from build123d import *

# Parameters (mm, degrees)
F0_W     = 12.85
F0_H     = 12.85
F0_W_2   = 6.2
F0_H_2   = 6.2
F1_DEPTH = 25
F2_DEPTH = 32.35
F3_SIZE  = 0.5
F4_SIZE  = 1


with BuildPart() as f1:
    # F0 (on Top) → F1 (new body)
    with BuildSketch(Plane.XY):
        Rectangle(F0_W, F0_H)
        Rectangle(F0_W_2, F0_H_2, mode=Mode.SUBTRACT)
    extrude(amount=F1_DEPTH)

    # F0 (on Top) → F2 (join)
    with BuildSketch(Plane.XY):
        Rectangle(F0_W_2, F0_H_2)
    extrude(amount=F2_DEPTH)

    # F3
    f3_edges = [f1.edges().sort_by_distance(p)[0] for p in [
        (3.1, -3.1, 28.675),
        (3.1, 3.1, 28.675),
        (-3.1, -3.1, 28.675),
        (-3.1, 3.1, 28.675),
        (-3.1, 0, 32.35),
        (0, 3.1, 32.35),
        (3.1, 0, 32.35),
        (0, -3.1, 32.35),
    ]]
    chamfer(f3_edges, length=F3_SIZE)

    # F4
    f4_edges = [f1.edges().sort_by_distance(p)[0] for p in [
        (-6.425, -6.425, 12.5),
        (-6.425, 6.425, 12.5),
        (6.425, 6.425, 12.5),
        (6.425, -6.425, 12.5),
    ]]
    chamfer(f4_edges, length=F4_SIZE)


solid = f1.part
Geometry check sheet. Reference: the model listing, model coordinates, mm. A direction names the side the tool comes from. Coordinates: 2 decimals unless noted, no trailing zeros. Loops run counter-clockwise (first coordinate to the right, second up) from the corner with the lowest first, then second, coordinate; pieces in that order, holes last. Notation, with made-up numbers: (26, -23.75) - (77, -23.75) arc R27 cw to (77, 2.25) - close; hole circle Ø4 at (-24, -19.75). An arc over 180 degrees is marked (long way). Use one line per item in the form item = value. Start each with the question number.
Item 1: Gauge pin test, flat ends, axial feed: pin 1 (1.6 mm diameter, centred on x = 0, z = 27.5, fed in from +Y); pin 2 (1.6 mm diameter, centred on y = -0.5, z = 27.5, fed in from -X); pin 3 (1.5 mm diameter, centred on x = -1.5, y = -3.5, fed in from +Z). Record the tip position at first contact, or that the pin passes through.
Item 2: Section check B-B, the plane x = -1.5. Enter the section's corners in (y, z) (3 decimals), and give its area (3 significant figures).
Item 3: Section check A-A, the plane z = 30. Enter the section's corners in (x, y).
Item 4: Tool access check on faces 1 (the face through (0, 3.1, 28)), 2 (the face through (0, -3.1, 28)), 3 (the face through (3.1, 0, 28)). Record the directions out of +Z, -Z, +X, -X, +Y, -Y that give a thin tool (end or side, any length) a straight path to the whole face; none if there is none.
Item 5: Thickness scan on probe 1 along Z at (x, y) = (-1, 5.75); probe 2 along X at (y, z) = (-0.75, 26); probe 3 along X at (y, z) = (5.5, 7). Record the ranges inside material, lowest first.
Item 6: Section check D-D, the plane y = -3.5. Enter the section's corners in (x, z) (3 decimals).
Computed:
q1.pin_1 = 3.1
q1.pin_2 = -3.1
q1.pin_3 = 32.2
q2.outline = (-6.425, 0) - (6.425, 0) - (6.425, 25) - (3.1, 25) - (3.1, 31.85) - (2.6, 32.35) - (-2.6, 32.35) - (-3.1, 31.85) - (-3.1, 25) - (-6.425, 25) - close
q2.area = 367 mm2
q3.outline = (-3.1, -2.6) - (-2.6, -3.1) - (2.6, -3.1) - (3.1, -2.6) - (3.1, 2.6) - (2.6, 3.1) - (-2.6, 3.1) - (-3.1, 2.6) - close
q4.face_1 = +Z, +X, -X, +Y
q4.face_2 = +Z, +X, -X, -Y
q4.face_3 = +Z, +X, +Y, -Y
q5.probe_1 = 0 to 25
q5.probe_2 = -3.1 to 3.1
q5.probe_3 = -6.35 to 6.35
q6.outline = (-6.425, 0) - (6.425, 0) - (6.425, 25) - (-6.425, 25) - close
